Could you check a few things on this model? Use its own coordinates, in mm. Give positions to 0.01 mm unless a question says otherwise; leave off trailing zeros. Write each loop counter-clockwise with the first axis right and the second up, starting at its lowest first coordinate (ties: lowest second). Pieces come first, ordered by that corner, then holes. Notation, with made-up numbers: (36.25, -2) - (67.25, -2) arc R30 ccw to (67.25, 28) - close; hole circle Ø8 at (88.25, 51). An arc over 180 degrees is marked (long way). Write item = value, one per line.
from build123d import *

# Parameters (mm, degrees)
SKETCH1_W           = 304.8
SKETCH1_H           = 609.6
BOSS_EXTRUDE1_DEPTH = 2.1082
CUT_EXTRUDE1_DEPTH  = 2.1082


with BuildPart() as part:
    # Sketch1 → Boss-Extrude1 (new body)
    with BuildSketch(Plane.XY):
        with Locations((101.6, -304.8)):
            Rectangle(SKETCH1_W, SKETCH1_H)
    extrude(amount=BOSS_EXTRUDE1_DEPTH)

    # Sketch2 → Cut-Extrude1 (cut)
    with BuildSketch(Plane.XY.offset(2.1082)):
        Polygon((-50.8, -609.6), (-50.8, -566.618355908), (0, -609.30496414), (156.491241029, -423.069623049), (181.170170025, -393.7), (254, -393.7), (254, -609.6), align=None)
    extrude(amount=-CUT_EXTRUDE1_DEPTH, mode=Mode.SUBTRACT)


solid = part.part
1. If we section it at B-B, the plane x = 189: Please give me the cut outline in (y, z), and give its area (3 significant figures).
Filled sheet:
outline = (-393.7, 0) - (0, 0) - (0, 2.11) - (-393.7, 2.11) - close
area = 830 mm2
2. If we section it at A-A, the plane z = 0.4: Please give me the cut outline in (x, y), and give its area (3 significant figures).
Filled sheet:
outline = (-50.8, -566.62) - (0, -609.3) - (181.17, -393.7) - (254, -393.7) - (254, 0) - (-50.8, 0) - close
area = 149,000 mm2
3. I need wall thicknesses on line 1 (X direction, y = -511, z = 1.95); line 2 (Y direction, x = 82, z = 1.35); line 3 (Y direction, x = 120, z = 1.7). Which ranges of each line are inside material? Lowest first, please.
Filled sheet:
line_1 = -50.8 to 82.6
line_2 = -511.72 to 0
line_3 = -466.5 to 0
4. If we section it at C-C, the plane y = -460.5: Please give me the cut outline in (x, z), and give its area (3 significant figures).
Filled sheet:
outline = (-50.8, 0) - (125.04, 0) - (125.04, 2.11) - (-50.8, 2.11) - close
area = 371 mm2
5. For pin 1 (0.6 mm diameter, centred on x = 220.5, z = 0.5, fed in from -Y), with a flat end and sliding along its axis, tell me the tip position at first contact or that it passes through.
Filled sheet:
pin_1 = -393.7
